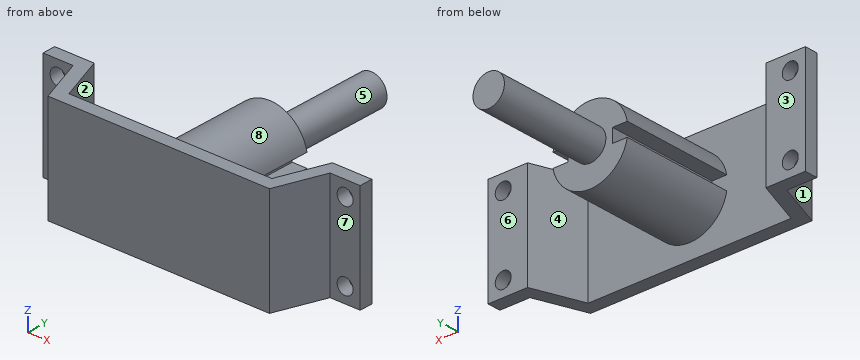
```python
from build123d import *

# Parameters (mm, degrees)
SKETCH1_W           = 50
SKETCH1_H           = 24
BOSS_EXTRUDE1_DEPTH = 3
BOSS_EXTRUDE2_DEPTH = 24
SKETCH3_R           = 8.525
BOSS_EXTRUDE3_DEPTH = 25.5
SKETCH4_R           = 3.55
BOSS_EXTRUDE4_DEPTH = 26
SKETCH5_W           = 4
SKETCH5_H           = 3.1
CUT_EXTRUDE1_DEPTH  = 25.5
CUT_EXTRUDE2_REACH  = 57.373
SKETCH6_R           = 1.8


with BuildPart() as part:
    # Sketch1 → Boss-Extrude1 (new body)
    with BuildSketch(Plane(origin=(0, 0, 0), x_dir=(1, 0, 0), z_dir=(0, 1, 0))):
        Rectangle(SKETCH1_W, SKETCH1_H)
    extrude(amount=BOSS_EXTRUDE1_DEPTH)

    # Sketch2 → Boss-Extrude2 (add)
    with BuildSketch(Plane.XY.offset(12)):
        Polygon((-25, 0), (-29.003672577, 11), (-35.803672577, 11), (-35.803672577, 14), (-26.903049962, 14), (-22.899377385, 3), align=None)
        Polygon((25, 0), (29.003672577, 11), (35.803672577, 11), (35.803672577, 14), (26.903049962, 14), (22.899377385, 3), align=None)
    extrude(amount=-BOSS_EXTRUDE2_DEPTH)

    # Sketch3 → Boss-Extrude3 (add)
    with BuildSketch(Plane(origin=(0, 3, 0), x_dir=(1, 0, 0), z_dir=(0, 1, 0))):
        with Locations(Location((0, 0, 0), (0, 0, 270))):
            Circle(SKETCH3_R)
    extrude(amount=BOSS_EXTRUDE3_DEPTH)

    # Sketch4 → Boss-Extrude4 (add)
    with BuildSketch(Plane(origin=(0, 28.5, 0), x_dir=(1, 0, 0), z_dir=(0, 1, 0))):
        with Locations(Location((0, 0, 0), (0, 0, 90))):
            Circle(SKETCH4_R)
    extrude(amount=BOSS_EXTRUDE4_DEPTH)

    # Sketch5 → Cut-Extrude1 (cut)
    with BuildSketch(Plane(origin=(0, 28.5, 0), x_dir=(1, 0, 0), z_dir=(0, 1, 0))):
        with Locations((-7.05, 0)):
            Rectangle(SKETCH5_W, SKETCH5_H)
        with Locations((7.05, 0)):
            Rectangle(SKETCH5_W, SKETCH5_H)
    extrude(amount=-CUT_EXTRUDE1_DEPTH, mode=Mode.SUBTRACT)

    # Sketch6 → Cut-Extrude2 (cut, up to next)
    with BuildSketch(Plane(origin=(0, 14, 0), x_dir=(1, 0, 0), z_dir=(0, 1, 0)), mode=Mode.PRIVATE) as cut_extrude2_sk1:
        with Locations(Location((-32.403672577, 8.6, 0), (0, 0, 270))):
            Circle(SKETCH6_R)
    cut_extrude2_tool1 = extrude(cut_extrude2_sk1.sketch, amount=-CUT_EXTRUDE2_REACH, mode=Mode.PRIVATE) & part.part
    # Sketch6 → Cut-Extrude2 (cut, up to next)
    with BuildSketch(Plane(origin=(0, 14, 0), x_dir=(1, 0, 0), z_dir=(0, 1, 0)), mode=Mode.PRIVATE) as cut_extrude2_sk2:
        with Locations((-32.403672577, -8.6)):
            Circle(SKETCH6_R)
    cut_extrude2_tool2 = extrude(cut_extrude2_sk2.sketch, amount=-CUT_EXTRUDE2_REACH, mode=Mode.PRIVATE) & part.part
    # Sketch6 → Cut-Extrude2 (cut, up to next)
    with BuildSketch(Plane(origin=(0, 14, 0), x_dir=(1, 0, 0), z_dir=(0, 1, 0)), mode=Mode.PRIVATE) as cut_extrude2_sk3:
        with Locations(Location((32.403672577, -8.6, 0), (0, 0, 270))):
            Circle(SKETCH6_R)
    cut_extrude2_tool3 = extrude(cut_extrude2_sk3.sketch, amount=-CUT_EXTRUDE2_REACH, mode=Mode.PRIVATE) & part.part
    # Sketch6 → Cut-Extrude2 (cut, up to next)
    with BuildSketch(Plane(origin=(0, 14, 0), x_dir=(1, 0, 0), z_dir=(0, 1, 0)), mode=Mode.PRIVATE) as cut_extrude2_sk4:
        with Locations((32.403672577, 8.6)):
            Circle(SKETCH6_R)
    cut_extrude2_tool4 = extrude(cut_extrude2_sk4.sketch, amount=-CUT_EXTRUDE2_REACH, mode=Mode.PRIVATE) & part.part
    add(cut_extrude2_tool1.solids().sort_by_distance((-32.403673, 14, -8.6))[0], mode=Mode.SUBTRACT)
    add(cut_extrude2_tool2.solids().sort_by_distance((-32.403673, 14, 8.6))[0], mode=Mode.SUBTRACT)
    add(cut_extrude2_tool3.solids().sort_by_distance((32.403673, 14, 8.6))[0], mode=Mode.SUBTRACT)
    add(cut_extrude2_tool4.solids().sort_by_distance((32.403673, 14, -8.6))[0], mode=Mode.SUBTRACT)


solid = part.part
```
Verification items for the finished model (mm, model axes). Face numbers are marked on the shaded views. A direction names the side the tool comes from. Give positions to 0.01 mm unless a question says otherwise; leave off trailing zeros. Loops run counter-clockwise (first coordinate to the right, second up) from the corner with the lowest first, then second, coordinate; pieces in that order, holes last. Notation, with made-up numbers: M 76,-25 L 121,-25 A25 ccw 121,13 Z; hole C -35.75,5.25 d8. An arc over 180 degrees is marked long. Return JSON: item names as keys, results as strings.
1) Section check C-C, the plane x = -2. Enter the section's corners in (y, z).
Findings:
{"outline": "M 0,-12 L 3,-12 L 3,-8.29 L 28.5,-8.29 L 28.5,-2.93 L 54.5,-2.93 L 54.5,2.93 L 28.5,2.93 L 28.5,8.29 L 3,8.29 L 3,12 L 0,12 Z"}
2) Section check D-D, the plane y = 17.5. Enter the section's corners in (x, z) (3 decimals), and give its area (3 significant figures).
Findings:
{"outline": "M -8.383,-1.55 A8.525 ccw 8.383,-1.55 L 5.05,-1.55 L 5.05,1.55 L 8.383,1.55 A8.525 ccw -8.383,1.55 L -5.05,1.55 L -5.05,-1.55 Z", "area": "207 mm2"}
3) Tool access check on the marked faces 4, 5, 6, 7 and 8. Record the directions out of +Z, -Z, +X, -X, +Y, -Y that give a thin tool (end or side, any length) a straight path to the whole face; none if there is none.
Findings:
{"face 4": "+Z, -Z, +Y", "face 5": "+Y", "face 6": "+Z, -Z, +X, +Y", "face 7": "+Z, -Z, +X, -Y", "face 8": "+Z, +Y"}
4) Gauge pin test, flat ends, axial feed: P1, Ø2.5, axis at x = 7, y = 9.5, coming from the +Z side; P2, Ø5.5, axis at x = 32.5, z = 5.5, coming from the -Y side; P3, Ø2.5, axis at x = -6, y = 17.5, coming from the -Z side. Record the tip position at first contact, or that the pin passes through.
Findings:
{"P1": "stops at z = 6.29", "P2": "stops at y = 11", "P3": "stops at z = -7.08"}
5) Section check A-A, the plane z = 7.75. Enter the section's corners in (x, y), and give its area (3 significant figures).
Findings:
{"outline": "M -35.8,11 L -33.99,11 L -33.99,14 L -35.8,14 Z; M -30.82,11 L -29,11 L -25,0 L 25,0 L 29,11 L 30.82,11 L 30.82,14 L 26.9,14 L 22.9,3 L 3.55,3 L 3.55,28.5 L -3.55,28.5 L -3.55,3 L -22.9,3 L -26.9,14 L -30.82,14 Z; M 33.99,11 L 35.8,11 L 35.8,14 L 33.99,14 Z", "area": "423 mm2"}
6) Material ranges on L1, parallel to X at y = 12.5, z = 4; L2, parallel to X at y = 13.1, z = 8.6; L3, parallel to X at y = 12.05, z = -8.6, recorded low to high. Write a range as [from, to].
Findings:
{"L1": "x = [-35.8, -26.36], [-7.53, 7.53], [26.36, 35.8]", "L2": "x = [-35.8, -34.2], [-30.6, -26.58], [26.58, 30.6], [34.2, 35.8]", "L3": "x = [-35.8, -34.2], [-30.6, -26.19], [26.19, 30.6], [34.2, 35.8]"}
7) Section check B-B, the plane z = 0. Enter the section's corners in (x, y), and give its area (3 significant figures).
Findings:
{"outline": "M -35.8,11 L -29,11 L -25,0 L 25,0 L 29,11 L 35.8,11 L 35.8,14 L 26.9,14 L 22.9,3 L 5.05,3 L 5.05,28.5 L 3.55,28.5 L 3.55,54.5 L -3.55,54.5 L -3.55,28.5 L -5.05,28.5 L -5.05,3 L -22.9,3 L -26.9,14 L -35.8,14 Z", "area": "703 mm2"}
8) Mould release check, pull along X, two halves, no side actions. Record for the marked faces 1, 2 and 3: released by +X, released by -X, zero draft, split by the parting line, or undercut.
Findings:
{"face 1": "released by -X", "face 2": "undercut", "face 3": "zero draft"}
